Geometry: final body of the model. Coordinates: model frame, mm. Face numbers are marked on the shaded views. A direction names the side the tool comes from. Round coordinates to 2 decimals unless told otherwise and drop trailing zeros. Order: outer loops, then holes, each group sorted by start corner. A loop starts at its lowest first (then second) coordinate and runs counter-clockwise, first axis right, second up. Notation, with made-up numbers: (5, 81) - (64, 81) arc R35 cw to (64, 117) - close; hole circle Ø3 at (-16, 53). An arc over 180 degrees is marked (long way). Put each result on its own line as item: value. Start each with the question number.
(1) Pull-direction query (Y, two-part tool) for the marked faces 4, 5 and 6; classes: released by +Y, released by -Y, zero draft, split by the parting line, or undercut.
(2) Section A-A (z = 16). Output: boundary loops of the cut face in (x, y).
(3) Material intervals for L1, parallel to Y at x = 0, z = -0.5; L2, parallel to Z at x = -31, y = 17; L3, parallel to Z at x = -3, y = 7.5, sorted ascending. Write a range as [from, to].
(4) Pin query (flat end, axial travel): P1, Ø6, axis at x = 19.5, y = -27, coming from the +Z side; P2, Ø6, axis at y = -18, z = 18, coming from the -X side; P3, Ø8, axis at x = 13.5, y = 28, coming from the -Z side. Return the tip coordinate at first contact, or that it passes through.
(5) Access query for the marked faces 1, 2 and 3. Directions: +Z, -Z, +X, -X, +Y, -Y. A direction counts if a zero-diameter tool reaches every point of the face in a straight line with its end or side. Return the directions, or none.
Autodesk Inventor part; units mm, degrees
ref_plane "YZ Plane" through (0, 0, 0) normal (1, 0, 0) x (0, 1, 0)
ref_plane "XZ Plane" through (0, 0, 0) normal (0, 1, 0) x (-1, 0, 0)
ref_plane "XY Plane" through (0, 0, 0) normal (0, 0, 1) x (1, 0, 0)
sketch "Esquisse1" plane through (0, 0, 0) normal (0, 0, 1) x (1, 0, 0)
  circle A0 centre (0, 0) radius 38.1
  circle A1 centre (0, 0) radius 2
  dimension "d0" = 76.2
  dimension "d1" = 4
extrude "Extrusion1" add sketch "Esquisse1" along normal blind 20
sketch "Esquisse2" plane through (0, 0, 20) normal (0, 0, 1) x (1, 0, 0)
  circle A0 centre (0, 0) radius 2
  circle A1 centre (0, 0) radius 38.1
  circle A2 centre (0, 0) radius 17.7233
extrude "Extrusion2" add sketch "Esquisse2" along normal blind 1 and the other way blind 21 contours A2
fillet "Congé1" radius 1 2 edges at (-38.1, 0, 20) (-38.1, 0, 0)
chamfer "Chanfrein1" distance 1 angle 45 2 edges at (-17.7233, 0, 20) (-17.7233, 0, 0)
sketch "Esquisse3" plane through (0, 0, -1) normal (0, 0, -1) x (-1, 0, 0)
  circle A0 centre (0, 0) radius 2
  circle A1 centre (0, 0) radius 17.7233
  circle A2 centre (0, 0) radius 16.7233
  circle A3 centre (0, 0) radius 3
  dimension "d12" = 1
  dimension "d13" = 1
extrude "Extrusion3" cut sketch "Esquisse3" against normal blind 1 contours A2
sketch "Esquisse4" plane through (0, 0, 21) normal (0, 0, 1) x (1, 0, 0)
  circle A0 centre (0, 0) radius 9.6
  circle A1 centre (0, 0) radius 2
  circle A2 centre (0, 0) radius 17.7233
  dimension "d16" = 19.2
extrude "Extrusion4" add sketch "Esquisse4" along normal blind 5.1 contours A0
sketch "Esquisse5" plane through (0, 0, 26.1) normal (0, 0, 1) x (1, 0, 0)
  circle A0 centre (0, 0) radius 2
  circle A1 centre (0, 0) radius 9.6
  circle A2 centre (0, 0) radius 6.05
  dimension "d19" = 12.1
extrude "Extrusion5" add sketch "Esquisse5" along normal blind 4.1 contours A2
properties part number "Roue"
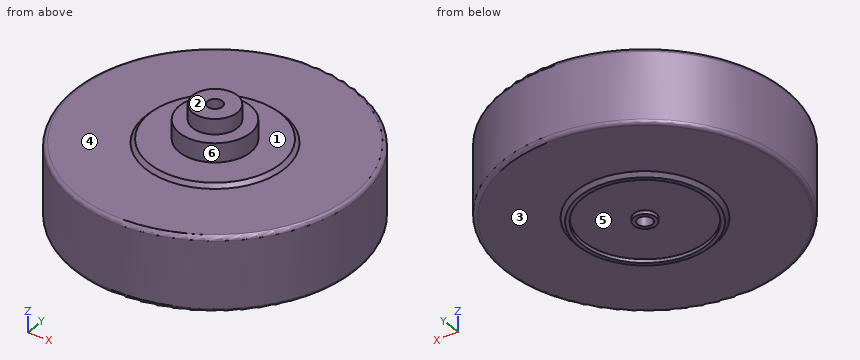
Checks:
1. face 4: zero draft
1. face 5: undercut
1. face 6: split by the parting line
2. outline: circle Ø76.2 at (0, 0); hole circle Ø4 at (0, 0)
3. L1: y = [-18.22, -16.72], [-3, -2], [2, 3], [16.72, 18.22]
3. L2: z = [0, 20]
3. L3: z = [0, 26.1]
4. P1: stops at z = 20
4. P2: stops at x = -35.02
4. P3: stops at z = 0
5. face 1: +Z
5. face 2: +Z, +X, -X, +Y, -Y
5. face 3: -Z
